For this review, use the dimensioned drawing (mm, ordinates from the lowest corner) and the shaded views. Give positions to 0.01 mm unless a question says otherwise; leave off trailing zeros. Order: outer loops, then holes, each group sorted by start corner. A loop starts at its lowest first (then second) coordinate and runs counter-clockwise, first axis right, second up.
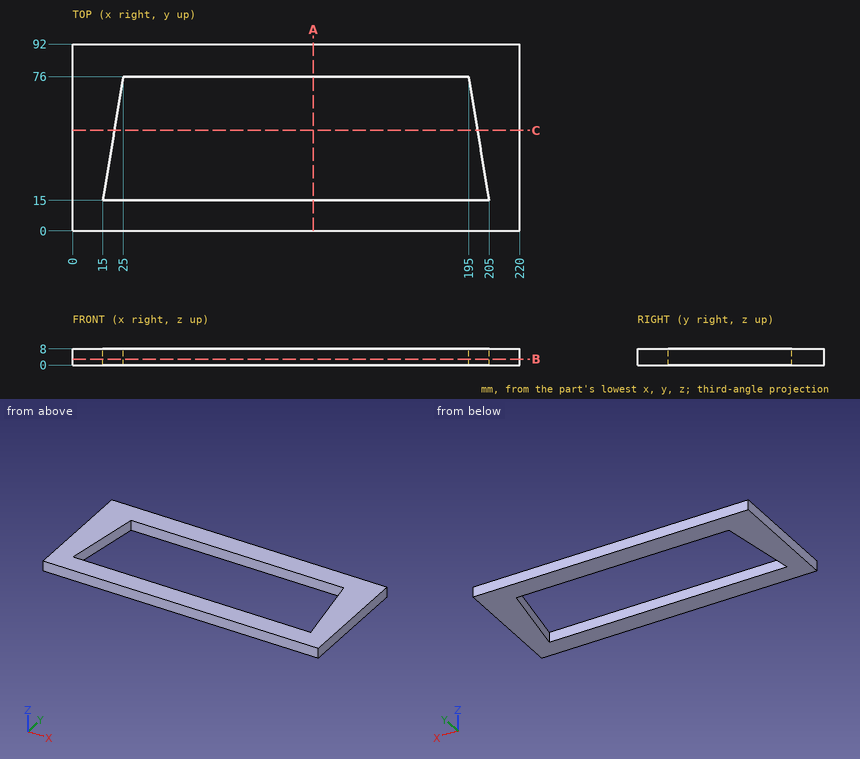
1. Take a section at A-A (x = 118.5). Write out the cut boundary in (y, z), and give its area (3 significant figures).
2. Take a section at C-C (y = 49.5). Write out the cut boundary in (x, z).
3. Insertion check: pin 1 (4 mm diameter, centred on x = 101, z = 5, fed in from -Y). The pin has a flat end and moves straight along its axis. Give the tip position at first contact, or say it passes through.
4. Take a section at B-B (z = 3). Write out the cut boundary in (x, y), and give its area (3 significant figures).
5. To check wall thickness, follow line 1 (Y direction, x = 169.5, z = 3.25); line 2 (X direction, y = 32, z = 1.5); line 3 (X direction, y = 21, z = 3.75). State the ranges of each line that lie inside material, in increasing order.
Answer:
1. outline: (0, 0) - (15, 0) - (15, 8) - (0, 8) - close; (76, 0) - (92, 0) - (92, 8) - (76, 8) - close
1. area: 248 mm2
2. outline: (0, 0) - (20.66, 0) - (20.66, 8) - (0, 8) - close; (199.34, 0) - (220, 0) - (220, 8) - (199.34, 8) - close
3. pin 1: stops at y = 0
4. outline: (0, 0) - (220, 0) - (220, 92) - (0, 92) - close; hole (15, 15) - (205, 15) - (195, 76) - (25, 76) - close
4. area: 9,260 mm2
5. line 1: y = 0 to 15, 76 to 92
5. line 2: x = 0 to 17.79, 202.21 to 220
5. line 3: x = 0 to 15.98, 204.02 to 220
